```python
from build123d import *

# Parameters (mm, degrees)
BOSS_EXTRUDE1_DEPTH     = 35.052
CUT_EXTRUDE1_DEPTH      = 231.935593134
CUT_EXTRUDE1_DEPTH_BACK = 231.935593134
SKETCH2_R               = 25.019
SKETCH2_R_2             = 10.033
CUT_EXTRUDE2_START      = -15.24
CUT_EXTRUDE2_DEPTH      = 15.24
FILLET1_R               = 9.906
SKETCH5_R               = 5.969
CUT_EXTRUDE3_DEPTH      = 231.935593134
CIRPATTERN1_COUNT       = 4
SKETCH6_W               = 250.475884559
SKETCH6_H               = 232.654927102
CUT_EXTRUDE4_DEPTH      = 20.066


with BuildPart() as part:
    # Sketch1 → Boss-Extrude1 (new body)
    with BuildSketch(Plane(origin=(0, 0, 0), x_dir=(1, 0, 0), z_dir=(0, 1, 0))):
        with BuildLine():
            Line((-14.986, 58.040528426), (97.409, 87.060792639))
            ThreePointArc((97.409, 87.060792639), (209.804, 0), (97.409, -87.060792639))
            Line((97.409, -87.060792639), (-14.986, -58.040528426))
            ThreePointArc((-14.986, -58.040528426), (-59.944, 0), (-14.986, 58.040528426))
        make_face()
    extrude(amount=BOSS_EXTRUDE1_DEPTH)

    # Sketch2 → Cut-Extrude1 (cut, two sides: drawn at the far end of the back side and taken through both)
    with BuildSketch(Plane(origin=(0, 35.052, 0), x_dir=(1, 0, 0), z_dir=(0, 1, 0)).offset(-CUT_EXTRUDE1_DEPTH_BACK)):
        with Locations(Location((119.888, 0, 0), (0, 0, 270))):
            Circle(SKETCH2_R)
        with Locations(Location((-30.226, 0, 0), (0, 0, 270))):
            Circle(SKETCH2_R_2)
    extrude(amount=CUT_EXTRUDE1_DEPTH + CUT_EXTRUDE1_DEPTH_BACK, mode=Mode.SUBTRACT)

    # Sketch3 → Cut-Extrude2 (cut)
    with BuildSketch(Plane(origin=(0, 35.052, 0), x_dir=(1, 0, 0), z_dir=(0, 1, 0)).offset(CUT_EXTRUDE2_START)):
        with BuildLine():
            ThreePointArc((-25.220705882, 54.380135443), (-59.944, 0), (-25.220705882, -54.380135443))
            ThreePointArc((-25.220705882, -54.380135443), (24.384, 0), (-25.220705882, 54.380135443))
        make_face()
    extrude(amount=CUT_EXTRUDE2_DEPTH, mode=Mode.SUBTRACT)

    # Fillet1
    # the kernel refuses this fillet: 9.906 mm, written as the material it takes off along each edge
    with BuildSketch(Plane(origin=(-25.220705882, 19.812, -54.380135443), x_dir=(0.9595509242122834, 0, -0.28153512008868975), z_dir=(0, 1, 0))) as fillet1_piece_1:
        with BuildLine():
            CenterArc((29.806229626, -9.900699967), FILLET1_R, 88.125665331, 131.182876807)
            Line((22.141504015, -16.176113683), (21.375031454, -16.803655054))
            ThreePointArc((21.375031454, -16.803655054), (11.518208373, -7.475588537), (-0.364835977, -0.92096855))
            Line((-0.364835977, -0.92096855), (-0.146921489, 0.979644035))
            ThreePointArc((-0.146921489, 0.979644035), (10.883650693, 1.620974317), (30.162629918, 0.990069997))
            Line((30.162629918, 0.990069997), (30.130229891, 0))
        make_face()
    extrude(amount=90.565574728, mode=Mode.SUBTRACT)
    with BuildSketch(Plane(origin=(-25.220705882, 19.812, 54.380135443), x_dir=(0.9595509242122835, 0, 0.2815351200886891), z_dir=(0, 1, 0))) as fillet1_piece_2:
        with BuildLine():
            CenterArc((29.806229626, 9.900699967), FILLET1_R, 140.691457861, 131.182876807)
            Line((22.141504015, 16.176113683), (21.375031454, 16.803655054))
            ThreePointArc((21.375031454, 16.803655054), (11.518208373, 7.475588537), (-0.364835977, 0.92096855))
            Line((-0.364835977, 0.92096855), (-0.146921489, -0.979644035))
            ThreePointArc((-0.146921489, -0.979644035), (10.883650693, -1.620974317), (30.162629918, -0.990069997))
            Line((30.162629918, -0.990069997), (30.130229891, 0))
        make_face()
    extrude(amount=90.565574728, mode=Mode.SUBTRACT)

    # Sketch5 → Cut-Extrude3 (cut, through all)
    with BuildSketch(Plane(origin=(0, 35.052, 0), x_dir=(1, 0, 0), z_dir=(0, 1, 0))):
        with Locations(Location((179.832, 0, 0), (0, 0, 270))):
            Circle(SKETCH5_R)
    cut_extrude3 = extrude(amount=-CUT_EXTRUDE3_DEPTH, mode=Mode.SUBTRACT)

    # CirPattern1: Cut-Extrude3 ×4 about axis
    cirpattern1_axis = Axis((119.888, 0, 0), (0, 1, 0))
    for i in range(1, CIRPATTERN1_COUNT):
        add(cut_extrude3.rotate(cirpattern1_axis, i * 360 / CIRPATTERN1_COUNT), mode=Mode.SUBTRACT)

    # Sketch6 → Cut-Extrude4 (cut)
    with BuildSketch(Plane.XZ):
        with Locations((165.115942279, 0)):
            Rectangle(SKETCH6_W, SKETCH6_H)
    extrude(amount=-CUT_EXTRUDE4_DEPTH, mode=Mode.SUBTRACT)


solid = part.part
```
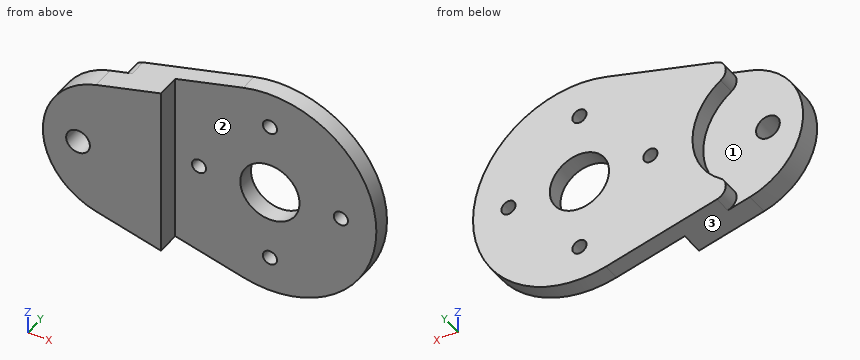
Design review of the part built by this model. Coordinates are the model's own, in mm. Face numbers are marked on the shaded views. Round coordinates to 2 decimals unless told otherwise and drop trailing zeros. Write each loop counter-clockwise with the first axis right and the second up, starting at its lowest first coordinate (ties: lowest second). Pieces come first, ordered by that corner, then holes.
Item 1: For probe 1 along X at (y, z) = (30, 0) (3 decimals); probe 2 along Y at (x, z) = (130, 32); probe 3 along Z at (x, y) = (-34, 9), list the stretches that pass through material, from the lowest coordinate up.
Item 2: We need section C-C on y = 9. Write out the cut boundary in (x, z), and give its area (3 significant figures).
Item 3: We need section B-B on y = 25.5. Write out the cut boundary in (x, z).
Item 4: Clearance check with flat-ended pins moving along their axes: pin 1 Ø3 at (x, y) = (37, 4.5) entering from -Z; pin 2 Ø2 at (y, z) = (10, 29) entering from -X; pin 3 Ø12 at (x, z) = (52.5, -62.5) entering from -Y. State where each tip first meets the part, or that it passes through.
Item 5: We need section D-D on z = 31.5. Write out the cut boundary in (x, y), and give its area (3 significant figures).
Item 6: We need section A-A on z = 0. Write out the cut boundary in (x, y) (3 decimals).
Item 7: The part is to be moulded in two halves that separate along Z. For the marked faces 1, 2 and 3, say which applies: +Z half, -Z half, draft (parallel to the pull), parting line (faces both ways), or undercut.
Returned:
1. probe 1: x = 24.384 to 53.975, 65.913 to 94.869, 144.907 to 173.863, 185.801 to 209.804
1. probe 2: y = 20.07 to 35.05
1. probe 3: z = -49.37 to -9.3, 9.3 to 49.37
2. outline: (-14.99, -58.04) - (39.88, -72.21) - (39.88, 72.21) - (-14.99, 58.04) arc R59.94 ccw to start; hole circle Ø20.07 at (-30.23, 0)
2. area: 10,700 mm2
3. outline: (0.58, -45.09) arc R9.91 ccw to (3.69, -62.86) - (97.41, -87.06) arc R89.92 ccw (long way) to (97.41, 87.06) - (3.69, 62.86) arc R9.91 ccw to (0.58, 45.09) arc R54.61 cw to start; hole circle Ø11.94 at (59.94, 0); hole circle Ø50.04 at (119.89, 0); hole circle Ø11.94 at (119.89, -59.94); hole circle Ø11.94 at (119.89, 59.94); hole circle Ø11.94 at (179.83, 0)
4. pin 1: stops at z = -71.85
4. pin 2: stops at x = -53
4. pin 3: stops at y = 20.07
5. outline: (-51, 0) - (39.88, 0) - (39.88, 20.07) - (204.11, 20.07) - (204.11, 35.05) - (14.38, 35.05) - (14.38, 19.81) - (-51, 19.81) - close
5. area: 4,650 mm2
6. outline: (-59.944, 0) - (-40.259, 0) - (-40.259, 19.812) - (-59.944, 19.812) - close; (-20.193, 0) - (39.878, 0) - (39.878, 20.066) - (53.975, 20.066) - (53.975, 35.052) - (24.384, 35.052) - (24.384, 19.812) - (-20.193, 19.812) - close; (65.913, 20.066) - (94.869, 20.066) - (94.869, 35.052) - (65.913, 35.052) - close; (144.907, 20.066) - (173.863, 20.066) - (173.863, 35.052) - (144.907, 35.052) - close; (185.801, 20.066) - (209.804, 20.066) - (209.804, 35.052) - (185.801, 35.052) - close
7. face 1: undercut
7. face 2: draft
7. face 3: -Z half
